Verification items for the finished model (mm, model axes). Round coordinates to 2 decimals unless told otherwise and drop trailing zeros. Loops run counter-clockwise (first coordinate to the right, second up) from the corner with the lowest first, then second, coordinate; pieces in that order, holes last. Notation, with made-up numbers: M 82,-6.75 L 118,-6.75 A24 ccw 118,14.25 Z; hole C -32.5,58.25 d11. An arc over 180 degrees is marked long. One line per item, written item: value.
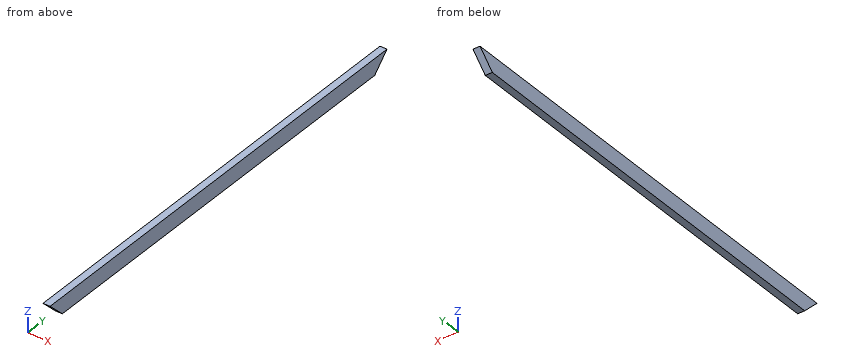
from build123d import *

# Parameters (mm, degrees)
F0_W     = 38.1
F0_H     = 88.9
F1_DEPTH = 1219.2
F2_SIZE2 = 88.89999
F2_SIZE  = 88.89999
F3_SIZE2 = 88.89999
F3_SIZE  = 88.89999


# Not quite as in the source:
# - a fillet or chamfer is up to 0.001 mm smaller than in the source, because OpenCascade refuses the exact size


with BuildPart() as f1:
    # F0 (on Front) → F1 (new body, symmetric)
    with BuildSketch(Plane.XZ):
        Rectangle(F0_W, F0_H)
    extrude(amount=F1_DEPTH, both=True)

    # F2 (size 88.9 and 88.9 in the source; OpenCascade refuses exactly that, so slightly less here)
    f2_edges = [f1.edges().sort_by_distance(p)[0] for p in [
        (0, -1219.2, -44.45),
    ]]
    chamfer(f2_edges, length=F2_SIZE, length2=F2_SIZE2)

    # F3 (size 88.9 and 88.9 in the source; OpenCascade refuses exactly that, so slightly less here)
    f3_edges = [f1.edges().sort_by_distance(p)[0] for p in [
        (0, 1219.2, -44.45),
    ]]
    chamfer(f3_edges, length=F3_SIZE, length2=F3_SIZE2)


solid = f1.part
(1) Sectioned sample at B-B on z = 11. Enter the section's corners in (x, y), and give its area (3 significant figures).
Completed:
outline: M -19.05,-1185.75 L 19.05,-1185.75 L 19.05,1185.75 L -19.05,1185.75 Z
area: 90,400 mm^2
(2) Thickness scan on L1, parallel to Y at x = -12.5, z = 11; L2, parallel to Y at x = -3.5, z = -29. Record the ranges inside material, lowest first. Write a range as from..to.
Completed:
L1: y = -1185.75..1185.75
L2: y = -1145.75..1145.75
(3) Depth check by flat-ended pin: pin 1 Ø10 at (x, z) = (-8, 2) entering from -Y; pin 2 Ø3 at (x, z) = (1, 0.5) entering from -Y; pin 3 Ø10 at (x, z) = (14, 29) entering from -Y. Enter the tip coordinate at first touch or a pass-through.
Completed:
pin 1: stops at y = -1181.75
pin 2: stops at y = -1176.75
pin 3: stops at y = -1208.75
